```python
from build123d import *

# Parameters (mm, degrees)
ESQUISSE1_R             = 20
BOSS_EXTRU_1_DEPTH      = 120
ESQUISSE3_R             = 16
ENL_V_MAT_EXTRU_1_DEPTH = 90
ENL_V_MAT_EXTRU_3_DEPTH = 140
ESQUISSE9_R             = 2
ENL_V_MAT_EXTRU_4_DEPTH = 10


with BuildPart() as part:
    # Esquisse1 → Boss.-Extru.1 (new body)
    with BuildSketch(Plane.XY):
        Circle(ESQUISSE1_R)
    extrude(amount=-BOSS_EXTRU_1_DEPTH)

    # Esquisse3 → Enlèv. mat.-Extru.1 (cut)
    with BuildSketch(Plane.XY.offset(-5)):
        Circle(ESQUISSE3_R)
    extrude(amount=-ENL_V_MAT_EXTRU_1_DEPTH, mode=Mode.SUBTRACT)

    # Esquisse6 → Enlèv. mat.-Extru.3 (cut)
    with BuildSketch(Plane(origin=(0, 0, -120), x_dir=(-1, 0, 0), z_dir=(0, 0, -1))):
        Polygon((-21.427885592, 0), (-21.427885592, -0.1), (22.282526064, -0.1), (22.282526064, 0.1), (-21.427885592, 0.1), align=None)
    extrude(amount=-ENL_V_MAT_EXTRU_3_DEPTH, mode=Mode.SUBTRACT)


with BuildPart() as body_2:
    # of the pieces the cut leaves, the one that is kept (enl_v_mat_extru_3_keep)
    add(part.part.solids().sort_by_distance((19.999749998, 0.1, 0))[0])

    # Esquisse8 → Enlèvement de matière-Révolution3 (revolve, cut)
    with BuildSketch(Plane.XZ.offset(-0.1)):
        with BuildLine():
            Line((-15.999687497, -95), (15.999687497, -95))
            ThreePointArc((15.999687497, -95), (0, -79.000312503), (-15.999687497, -95))
        make_face()
    revolve(axis=Axis((-15.999687497, 0.1, -95), (1, 0, 0)), mode=Mode.SUBTRACT)

    # Esquisse9 → Enlèv. mat.-Extru.4 (cut)
    with BuildSketch(Plane.XY):
        Circle(ESQUISSE9_R)
    extrude(amount=-ENL_V_MAT_EXTRU_4_DEPTH, mode=Mode.SUBTRACT)


solid = body_2.part
```
Geometry: final body of the model. Coordinates: model frame, mm. A direction names the side the tool comes from. Give positions to 0.01 mm unless a question says otherwise; leave off trailing zeros. Order: outer loops, then holes, each group sorted by start corner. A loop starts at its lowest first (then second) coordinate and runs counter-clockwise, first axis right, second up. Notation, with made-up numbers: (2.5, -28.75) -> (23.5, -28.75) arc R21 cw to (23.5, 10.25) -> close; hole circle Ø5 at (48.25, -23.5). An arc over 180 degrees is marked (long way). Write each question's results on one line, items separated by ' | '. Start each with the question number.
1) Section A-A (x = 0). Return loops of the section in (y, z), then the cut area to 3 significant figures.
2) Section D-D (y = 3.25). Return loops of the section in (x, z), then the cut area to 3 significant figures.
3) First-contact query: pin 1 (8 mm diameter, centred on x = 5.5, z = -93, fed in from +Y); pin 2 (8 mm diameter, centred on x = 2.5, z = -101, fed in from -Y); pin 3 (2 mm diameter, centred on y = 8.5, z = -59.5, fed in from -X). Flat tips, straight axial feed; report the tip coordinate or a pass-through.
4) Section C-C (z = -22). Return loops of the section in (x, y), then the cut area to 3 significant figures.
5) Section B-B (y = 13.75). Return loops of the section in (x, z).
6) Set-up query: faces 4 (the flat face through (0, 8, 0)), 5 (the cylindrical face through (0, 2, -2)), 6 (the cylindrical face through (0, 16, -49)). Return all of +Z, -Z, +X, -X, +Y, -Y with unobstructed straight access to the full face (end or side cutting, diameter ignored); none if empty.
7) Draft query along X for faces 1 (the flat face through (0, 6, -5)), 2 (the cylindrical face through (0, 20, -59)), 3 (the flat face through (16.2, 0.1, -73.6)). Return one class per face: pulls with the +X half, pulls with the -X half, needs draft (parallel to the pull), parting line crosses it, or undercut.
8) Line query: line 1 (X direction, y = 7.25, z = -107.5); line 2 (Z direction, x = -3.5, y = 8); line 3 (Z direction, x = -10.5, y = 8.5). Output: solid intervals per line, ascending. Write a range as from..to.
Calculated:
1) outline: (0.1, -120) -> (20, -120) -> (20, 0) -> (2, 0) -> (2, -5) -> (16, -5) -> (16, -93.22) arc R16 cw to (0.1, -111) -> close | area: 746 mm2
2) outline: (-19.73, -120) -> (19.73, -120) -> (19.73, 0) -> (-19.73, 0) -> close; hole (-15.67, -94.21) arc R15.69 ccw (long way) to (15.67, -94.21) -> (15.67, -5) -> (-15.67, -5) -> close | area: 1,530 mm2
3) pin 1: y = 19.94 | pin 2: y = 12.17 | pin 3: x = -18.54
4) outline: (-20, 0.1) -> (-16, 0.1) arc R16 cw to (16, 0.1) -> (20, 0.1) arc R20 ccw to start | area: 225 mm2
5) outline: (-14.52, -120) -> (14.52, -120) -> (14.52, 0) -> (-14.52, 0) -> close; hole (-8.18, -93.35) arc R8.35 ccw (long way) to (8.18, -93.35) -> (8.18, -5) -> (-8.18, -5) -> close
6) face 4: +Z, +X, -X, +Y, -Y | face 5: +Z, -Y | face 6: -Y
7) face 1: undercut | face 2: parting line crosses it | face 3: needs draft
8) line 1: -18.64..-6.97, 6.97..18.64 | line 2: -120..-108.47, -5..0 | line 3: -120..-103.67, -5..0
